Verification items for the finished model (mm, model axes). Face numbers are marked on the shaded views. Coordinates: 2 decimals unless noted, no trailing zeros. Order: outer loops, then holes, each group sorted by start corner. A loop starts at its lowest first (then second) coordinate and runs counter-clockwise, first axis right, second up.
Q1. Thickness scan on line 1 (Y direction, x = 0, z = 10.15); line 2 (Z direction, x = 0.75, y = -175); line 3 (X direction, y = -120, z = -2.5). Record the ranges inside material, lowest first.
Q2. Cross-section at A-A, the plane x = 5.5. Record the boundary of the cut face in (y, z).
Q3. Depth check by flat-ended pin: P1, Ø3, axis at x = 7, y = -89, coming from the +Z side; P2, Ø1.3, axis at y = -24.5, z = 10, coming from the -X side; P3, Ø0.5, axis at y = -38.5, z = -10, coming from the +X side; P4, Ø10, axis at x = 1.5, z = 0.5, coming from the +Y side. Enter the tip coordinate at first touch or a pass-through.
Q4. Cross-section at D-D, the plane x = -7.25. Record the boundary of the cut face in (y, z), and give its area (3 significant figures).
Q5. Draft check along Z on the marked faces 1 and 2. Enter one of: pulls with the +Z half, pulls with the -Z half, needs draft (parallel to the pull), parting line crosses it, or undercut.
from build123d import *

# Parameters (mm, degrees)
F0_R     = 11.1125
F0_R_2   = 9.525
F1_DEPTH = 212.852
F2_R     = 2.38125
F2_R_2   = 3.175
F2_R_3   = 1.5875
F3_DEPTH = 25.4
F4_R     = 1.27
F4_R_2   = 3.175
F5_DEPTH = 25.4


with BuildPart() as f1:
    # F0 (on Front) → F1 (new body)
    with BuildSketch(Plane.XZ):
        Circle(F0_R)
        Circle(F0_R_2, mode=Mode.SUBTRACT)
    extrude(amount=F1_DEPTH)

    # F2 (on Top) → F3 (cut)
    with BuildSketch(Plane.XY):
        with Locations((0, -4.7625)):
            Circle(F2_R)
        with BuildLine():
            ThreePointArc((-2.38125, -50.8), (0, -53.18125), (2.38125, -50.8))
            Line((2.38125, -50.8), (2.38125, -31.75))
            ThreePointArc((2.38125, -31.75), (0, -29.36875), (-2.38125, -31.75))
            Line((-2.38125, -31.75), (-2.38125, -50.8))
        make_face()
        with Locations((0, -69.85)):
            Circle(F2_R_2)
        with Locations((0, -79.375)):
            Circle(F2_R_2)
        with Locations((0, -123.825)):
            Circle(F2_R_3)
    extrude(amount=-F3_DEPTH, mode=Mode.SUBTRACT)

    # F4 (on Top) → F5 (cut)
    with BuildSketch(Plane.XY):
        with BuildLine():
            ThreePointArc((2.032, -6.004002), (2.292275, -5.407346), (2.38125, -4.7625))
            ThreePointArc((2.38125, -4.7625), (-0.644846, -2.470225), (-2.032, -6.004002))
            ThreePointArc((-2.032, -6.004002), (0, -7.14375), (2.032, -6.004002))
        make_face()
        with BuildLine():
            ThreePointArc((2.032, -6.004002), (0, -7.14375), (-2.032, -6.004002))
            Line((-2.032, -6.004002), (-2.032, -39.6875))
            Line((-2.032, -39.6875), (0, -39.6875))
            Line((0, -39.6875), (2.032, -39.6875))
            Line((2.032, -39.6875), (2.032, -6.004002))
        make_face()
        with BuildLine():
            Line((0, -39.6875), (-2.032, -39.6875))
            ThreePointArc((-2.032, -39.6875), (0, -41.700798), (2.032, -39.6875))
            Line((2.032, -39.6875), (0, -39.6875))
        make_face()
        with Locations((0, -57.15)):
            Circle(F4_R)
        with Locations((0, -68.2625)):
            Circle(F4_R)
        with Locations((0, -79.375)):
            Circle(F4_R_2)
    extrude(amount=F5_DEPTH, mode=Mode.SUBTRACT)


solid = f1.part
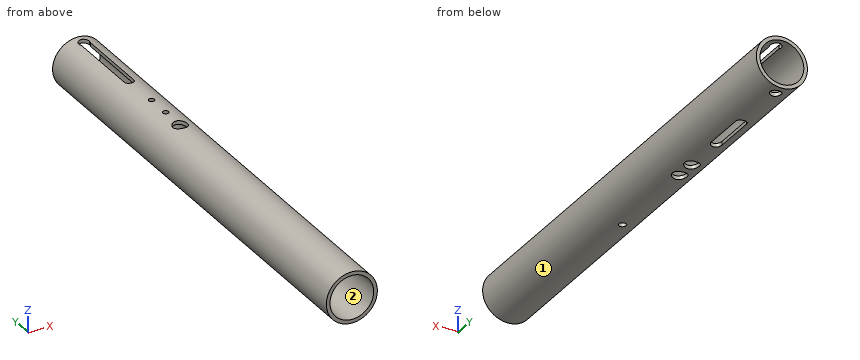
Check values:
1. line 1: y = -212.85 to -82.55, -76.2 to -69.53, -66.99 to -58.42, -55.88 to -41.7, -2.38 to 0
1. line 2: z = -11.09 to -9.5, 9.5 to 11.09
1. line 3: x = -10.83 to -9.19, 9.19 to 10.83
2. outline: (-212.85, -9.66) - (0, -9.66) - (0, -7.78) - (-212.85, -7.78) - close; (-212.85, 7.78) - (0, 7.78) - (0, 9.66) - (-212.85, 9.66) - close
3. P1: stops at z = 9.66
3. P2: stops at x = -6.01
3. P3: stops at x = 5.33
3. P4: passes through
4. outline: (-212.85, -8.42) - (0, -8.42) - (0, -6.18) - (-212.85, -6.18) - close; (-212.85, 6.18) - (0, 6.18) - (0, 8.42) - (-212.85, 8.42) - close
4. area: 955 mm2
5. face 1: parting line crosses it
5. face 2: undercut
